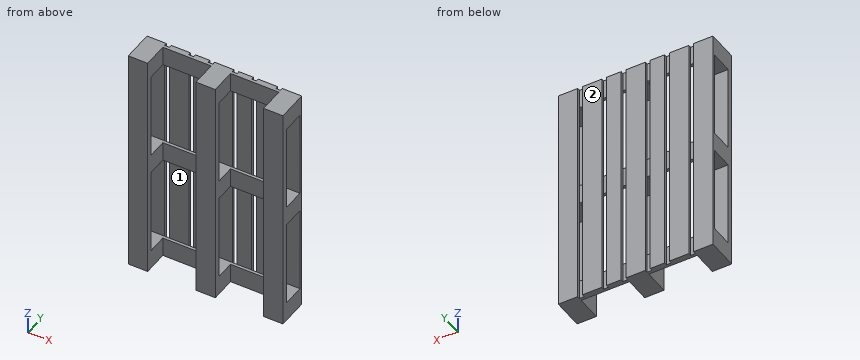
```python
from build123d import *

# Parameters (mm, degrees)
SKETCH1_W              = 800
SKETCH1_H              = 1200
BOSS_EXTRUDE2_DEPTH    = 160
CUT_EXTRUDE2_START     = -800
CUT_EXTRUDE2_OUTLINE_W = 450
CUT_EXTRUDE2_OUTLINE_H = 115
CUT_EXTRUDE2_DEPTH     = 800
SKETCH4_W              = 250
SKETCH4_H              = 130
CUT_EXTRUDE3_DEPTH     = 1452.068571777
SKETCH6_W              = 25
SKETCH6_H              = 1200
CUT_EXTRUDE5_DEPTH     = 15


# Read off the part's stored shape, not the designer's step: Cut-Extrude2
with BuildPart() as part:
    # Sketch1 → Boss-Extrude2 (new body)
    with BuildSketch(Plane(origin=(0, 0, 0), x_dir=(1, 0, 0), z_dir=(0, 1, 0))):
        with Locations((-400, 600)):
            Rectangle(SKETCH1_W, SKETCH1_H)
    extrude(amount=BOSS_EXTRUDE2_DEPTH)

    # Cut-Extrude2 outline → Cut-Extrude2 (cut)
    with BuildSketch(Plane.ZY.offset(800).offset(CUT_EXTRUDE2_START)):
        with Locations((-325, 87.5)):
            Rectangle(CUT_EXTRUDE2_OUTLINE_W, CUT_EXTRUDE2_OUTLINE_H)
        with Locations((-875, 87.5)):
            Rectangle(CUT_EXTRUDE2_OUTLINE_W, CUT_EXTRUDE2_OUTLINE_H)
    extrude(amount=CUT_EXTRUDE2_DEPTH, mode=Mode.SUBTRACT)

    # Sketch4 → Cut-Extrude3 (cut, through all)
    with BuildSketch(Plane.XY):
        with Locations((-575, 65)):
            Rectangle(SKETCH4_W, SKETCH4_H)
        with Locations((-225, 65)):
            Rectangle(SKETCH4_W, SKETCH4_H)
    extrude(amount=-CUT_EXTRUDE3_DEPTH, mode=Mode.SUBTRACT)

    # Sketch6 → Cut-Extrude5 (cut)
    with BuildSketch(Plane(origin=(0, 160, 0), x_dir=(1, 0, 0), z_dir=(0, 1, 0))):
        with Locations((-687.5, 600)):
            Rectangle(SKETCH6_W, SKETCH6_H)
        with Locations((-462.5, 600)):
            Rectangle(SKETCH6_W, SKETCH6_H)
        with Locations((-562.5, 600)):
            Rectangle(SKETCH6_W, SKETCH6_H)
        with Locations((-337.5, 600)):
            Rectangle(SKETCH6_W, SKETCH6_H)
        with Locations((-112.5, 600)):
            Rectangle(SKETCH6_W, SKETCH6_H)
        with Locations((-237.5, 600)):
            Rectangle(SKETCH6_W, SKETCH6_H)
    extrude(amount=-CUT_EXTRUDE5_DEPTH, mode=Mode.SUBTRACT)


solid = part.part
```
Could you check a few things on this model? Use its own coordinates, in mm. Face numbers are marked on the shaded views. A direction names the side the tool comes from. Round coordinates to 2 decimals unless told otherwise and drop trailing zeros. Order: outer loops, then holes, each group sorted by start corner. A loop starts at its lowest first (then second) coordinate and runs counter-clockwise, first axis right, second up. Notation, with made-up numbers: (77, -14.5) -> (125, -14.5) arc R14 cw to (125, 3.5) -> close; hole circle Ø5 at (30, 0.5). An arc over 180 degrees is marked (long way). One line per question, with ' | ' between items.
Q1. I'm going to push flat-ended pins straight in: pin 1 (22.5 mm diameter, centred on x = -294, z = -428, fed in from -Y); pin 2 (7.5 mm diameter, centred on x = -561, z = -1128.5, fed in from +Y). Where does each tip first touch, or does it pass through?
Computed values:
pin 1: y = 145 | pin 2: y = 145
Q2. If we section it at B-B on y = 63: Give the number of separate pieces and of enclosed holes in the cut face, plus the area to 3 significant figures.
Computed values:
separate pieces: 9 | enclosed holes: 0 | area: 90,000 mm²
Q3. If I drill on line 1 (X direction, y = 85, z = -649); line 2 (Z direction, x = -440, y = 47.5); line 3 (Y direction, x = -446, z = -505), over which ranges is the centre line in solid material (lowest first)? Write a range as from..to.
Computed values:
line 1: -800..-700, -450..-350, -100..0 | line 2: -1200..-1100, -650..-550, -100..0 | line 3: 0..30, 145..160
Q4. If we section it at A-A on x = -373: Write out the boundary of the cut face in (y, z), plus the area to 3 significant figures.
Computed values:
outline: (0, -1200) -> (160, -1200) -> (160, 0) -> (0, 0) -> close; hole (30, -1100) -> (145, -1100) -> (145, -650) -> (30, -650) -> close; hole (30, -550) -> (145, -550) -> (145, -100) -> (30, -100) -> close | area: 88,500 mm²
Q5. Which directions (+Z, -Z, +X, -X, +Y, -Y) give clear straight access to the entire face, cutting with the end or side of a thin tool? Please do the marked faces 1 and 2.
Computed values:
face 1: +X, -X, -Y | face 2: +Z, -Z, +X, -X, +Y
Q6. If we section it at D-D on x = -183: Write out the boundary of the cut face in (y, z).
Computed values:
outline: (130, -1200) -> (160, -1200) -> (160, 0) -> (130, 0) -> (130, -100) -> (145, -100) -> (145, -550) -> (130, -550) -> (130, -650) -> (145, -650) -> (145, -1100) -> (130, -1100) -> close
